Input: part model. Units: mm. Frame: model coordinates. Round coordinates to 2 decimals unless told otherwise and drop trailing zeros. Write each loop counter-clockwise with the first axis right and the second up, starting at its lowest first coordinate (ties: lowest second). Pieces come first, ordered by that corner, then holes. Notation, with made-up numbers: (-14.5, 32) -> (-4.5, 32) arc R35 ccw to (-4.5, 71) -> close; hole circle Ø11 at (-10, 82). An arc over 180 degrees is marked (long way). Write item = value, one per line. Start each with the question number.
```python
from build123d import *

# Parameters (mm, degrees)
SKETCH_1_R      = 11
SKETCH_1_R_2    = 1.1
EXTRUDE_1_DEPTH = 22


with BuildPart() as part:
    # 草图1 → 凸台-拉伸1 (new body)
    with BuildSketch(Plane.XY):
        Circle(SKETCH_1_R)
        with Locations((0, 7.5)):
            Circle(SKETCH_1_R_2, mode=Mode.SUBTRACT)
        with Locations((0, -7.5)):
            Circle(SKETCH_1_R_2, mode=Mode.SUBTRACT)
        with Locations((-6.495190528, -3.75)):
            Circle(SKETCH_1_R_2, mode=Mode.SUBTRACT)
        with Locations(Location((6.495190528, -3.75, 0), (0, 0, 180))):
            Circle(SKETCH_1_R_2, mode=Mode.SUBTRACT)
    extrude(amount=EXTRUDE_1_DEPTH)


solid = part.part
```
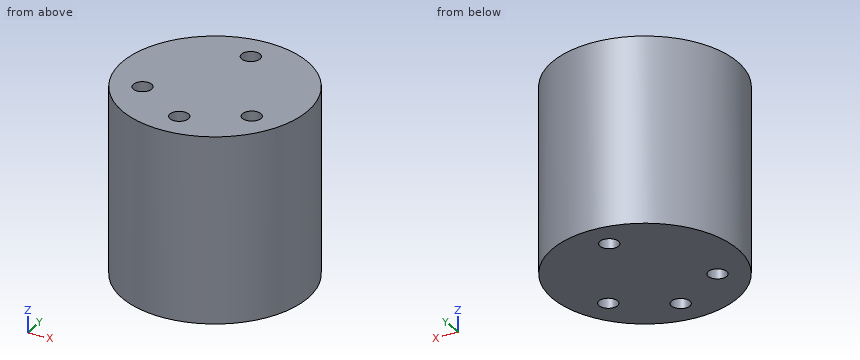
1. Section B-B (z = 2.75). Output: boundary loops of the cut face in (x, y).
2. Section D-D (x = 6.25). Output: boundary loops of the cut face in (y, z), then the cut area to 3 significant figures.
3. Pin query (flat end, axial travel): P1, Ø5, axis at y = 8, z = 11.5, coming from the +X side; P2, Ø6, axis at y = 7.5, z = 14.5, coming from the +X side; P3, Ø1, axis at y = 5.5, z = 16.5, coming from the +X side. Return the tip coordinate at first contact, or that it passes through.
4. Section C-C (y = 7.5). Output: boundary loops of the cut face in (x, z), then the cut area to 3 significant figures.
5. Line query: line 1 along Y through (x, z) = (0, 7.75); line 2 along Y through (x, z) = (1, 8); line 3 along X through (y, z) = (-2.75, 18.5). Output: solid intervals per line, ascending.
6. Section A-A (x = 0). Output: boundary loops of the cut face in (y, z), then the cut area to 3 significant figures.
Check sheet entries:
q1.outline = circle Ø22 at (0, 0); hole circle Ø2.2 at (-6.5, -3.75); hole circle Ø2.2 at (0, -7.5); hole circle Ø2.2 at (0, 7.5); hole circle Ø2.2 at (6.5, -3.75)
q2.outline = (-9.05, 0) -> (-4.82, 0) -> (-4.82, 22) -> (-9.05, 22) -> close; (-2.68, 0) -> (9.05, 0) -> (9.05, 22) -> (-2.68, 22) -> close
q2.area = 351 mm2
q3.P1 = 9.53
q3.P2 = 10.04
q3.P3 = 9.8
q4.outline = (-8.05, 0) -> (-1.1, 0) -> (-1.1, 22) -> (-8.05, 22) -> close; (1.1, 0) -> (8.05, 0) -> (8.05, 22) -> (1.1, 22) -> close
q4.area = 306 mm2
q5.line_1 = -11 to -8.6, -6.4 to 6.4, 8.6 to 11
q5.line_2 = -10.95 to -7.96, -7.04 to 7.04, 7.96 to 10.95
q5.line_3 = -10.65 to -6.95, -6.04 to 6.04, 6.95 to 10.65
q6.outline = (-11, 0) -> (-8.6, 0) -> (-8.6, 22) -> (-11, 22) -> close; (-6.4, 0) -> (6.4, 0) -> (6.4, 22) -> (-6.4, 22) -> close; (8.6, 0) -> (11, 0) -> (11, 22) -> (8.6, 22) -> close
q6.area = 387 mm2
